For this review, take the finished solid that the model builds, in its own axes (mm). A direction names the side the tool comes from. Give positions to 0.01 mm unless a question says otherwise; leave off trailing zeros. Order: outer loops, then holes, each group sorted by start corner. A loop starts at its lowest first (then second) coordinate and runs counter-clockwise, first axis right, second up. Notation, with made-up numbers: M 9.5,26.5 L 30.5,26.5 A20 ccw 30.5,31.5 Z; hole C -35.75,4 d5. An arc over 180 degrees is marked long. Use CSV: the item, a comma, the result in double quotes. Start each with the question number.
(1) Consider section B-B (x = 44.5). Write out the cut boundary in (y, z), and give its area (3 significant figures).
(2) Consider section D-D (z = 0). Write out the cut boundary in (x, y).
(3) Clearance check with flat-ended pins moving along their axes: P1, Ø3, axis at x = -29, z = 2.5, coming from the +Y side; P2, Ø7, axis at x = -10, z = 24, coming from the +Y side; P3, Ø5, axis at x = -42.5, y = 52.5, coming from the -Z side. State where each tip first meets the part, or that it passes through.
(4) Consider section A-A (y = 78). Write out the cut boundary in (x, z).
(5) Consider section C-C (y = 67). Write out the cut boundary in (x, z).
(6) Wall thickness on L1, parallel to Z at x = 44.5, y = 89; L2, parallel to Z at x = 3.5, y = 31.5; L3, parallel to Y at x = 24, z = -18: over which ranges is each line inside the solid? List them lowest first. Write a range as from..to.
(7) Tool access review of faces 1 (the face through (29, 76, 0)), 2 (the face through (-1, 5, -23)), 3 (the face through (45, 73, 0)), 4 (the face through (-1, 5, 23)): name each direction out of +Z, -Z, +X, -X, +Y, -Y from which nothing blocks a thin tool from reaching the whole face with its end or side.
(8) Draft analysis for pull direction Z (two halves, no side actions). For faces 5 (the face through (-1, 0, -30)), 6 (the face through (47.7, 84.2, -2.4)), 7 (the face through (-31, 86, 0)), 8 (the face through (1, 47, 6.5)), state which applies: pulls with the +Z half, pulls with the -Z half, needs draft (parallel to the pull), parting line crosses it, or undercut.
```python
from build123d import *

# Parameters (mm, degrees)
SKETCH1_W           = 108
SKETCH1_H           = 10
BOSS_EXTRUDE1_DEPTH = 30
BOSS_EXTRUDE2_DEPTH = 6.5
SKETCH3_R           = 4
CUT_EXTRUDE1_DEPTH  = 22
FILLET1_R           = 10


with BuildPart() as part:
    # Sketch1 → Boss-Extrude1 (new, symmetric)
    with BuildSketch(Plane.XY):
        Rectangle(SKETCH1_W, SKETCH1_H)
    extrude(amount=BOSS_EXTRUDE1_DEPTH, both=True)

    # Sketch2 → Boss-Extrude2 (add, symmetric)
    with BuildSketch(Plane.XY):
        with BuildLine():
            Line((-54, 5), (-54, 95))
            Line((-54, 95), (-31, 95))
            Line((-31, 95), (-31, 76))
            Line((-31, 76), (-27.5, 76))
            ThreePointArc((-27.5, 76), (0, 48.5), (27.5, 76))
            Line((27.5, 76), (31, 76))
            Line((31, 76), (31, 95))
            Line((31, 95), (54, 95))
            Line((54, 95), (54, 5))
            Line((54, 5), (-54, 5))
        make_face()
    extrude(amount=BOSS_EXTRUDE2_DEPTH, both=True)

    # Sketch3 → Cut-Extrude1 (cut)
    with BuildSketch(Plane(origin=(0, 95, 0), x_dir=(1, 0, 0), z_dir=(0, 1, 0))):
        with Locations(Location((44.5, 0, 0), (0, 0, 180))):
            Circle(SKETCH3_R)
        with Locations((-43.715454096, 0)):
            Circle(SKETCH3_R)
    extrude(amount=-CUT_EXTRUDE1_DEPTH, mode=Mode.SUBTRACT)

    # Fillet1
    fillet1_edges = [part.edges().sort_by_distance(p)[0] for p in [
        (0, 5, -6.5),
        (0, 5, 6.5),
    ]]
    fillet(fillet1_edges, radius=FILLET1_R)


solid = part.part
```
Check result:
1,outline,"M -5,-30 L 5,-30 L 5,-16.5 A10 cw 15,-6.5 L 95,-6.5 L 95,-4 L 73,-4 L 73,4 L 95,4 L 95,6.5 L 15,6.5 A10 cw 5,16.5 L 5,30 L -5,30 Z"
1,area,"1,640 mm^2"
2,outline,"M -54,-5 L 54,-5 L 54,95 L 48.5,95 L 48.5,73 L 40.5,73 L 40.5,95 L 31,95 L 31,76 L 27.5,76 A27.5 cw -27.5,76 L -31,76 L -31,95 L -39.72,95 L -39.72,73 L -47.72,73 L -47.72,95 L -54,95 Z"
3,P1,"stops at y = 76"
3,P2,"stops at y = 5"
3,P3,"stops at z = -6.5"
4,outline,"M -54,-6.5 L -31,-6.5 L -31,6.5 L -54,6.5 Z; M 31,-6.5 L 54,-6.5 L 54,6.5 L 31,6.5 Z; hole C -43.72,0 d8; hole C 44.5,0 d8"
5,outline,"M -54,-6.5 L -25.99,-6.5 L -25.99,6.5 L -54,6.5 Z; M 25.99,-6.5 L 54,-6.5 L 54,6.5 L 25.99,6.5 Z"
6,L1,"z = -6.5..-4, 4..6.5"
6,L2,"z = -6.5..6.5"
6,L3,"y = -5..5"
7,face 1,"+Z, -Z, +Y"
7,face 2,"-Z, +X, -X, +Y"
7,face 3,"+Y"
7,face 4,"+Z, +X, -X, +Y"
8,face 5,"pulls with the -Z half"
8,face 6,"undercut"
8,face 7,"needs draft"
8,face 8,"pulls with the +Z half"
